from build123d import *

# Parameters (mm, degrees)
SKETCH1_W    = 139.7
SKETCH1_H    = 9.53
BLOCK1_DEPTH = 71.42
SKETCH2_W    = 9.53
SKETCH2_H    = 38.1
BLOCK2_DEPTH = 71.42
SKETCH3_W    = 9.53
SKETCH3_H    = 38.1
BLOCK3_DEPTH = 71.42


with BuildPart() as part:
    # Sketch1 → Block1 (new body)
    with BuildSketch(Plane.XY.offset(-35.71)):
        with Locations((0, 4.765)):
            Rectangle(SKETCH1_W, SKETCH1_H)
    extrude(amount=BLOCK1_DEPTH)

    # Sketch2 → Block2 (add)
    with BuildSketch(Plane.XY.offset(-35.71)):
        with Locations((-55.565, 28.58)):
            Rectangle(SKETCH2_W, SKETCH2_H)
    extrude(amount=BLOCK2_DEPTH)

    # Sketch3 → Block3 (add)
    with BuildSketch(Plane.XY.offset(-35.71)):
        with Locations((55.565, 28.58)):
            Rectangle(SKETCH3_W, SKETCH3_H)
    extrude(amount=BLOCK3_DEPTH)


solid = part.part
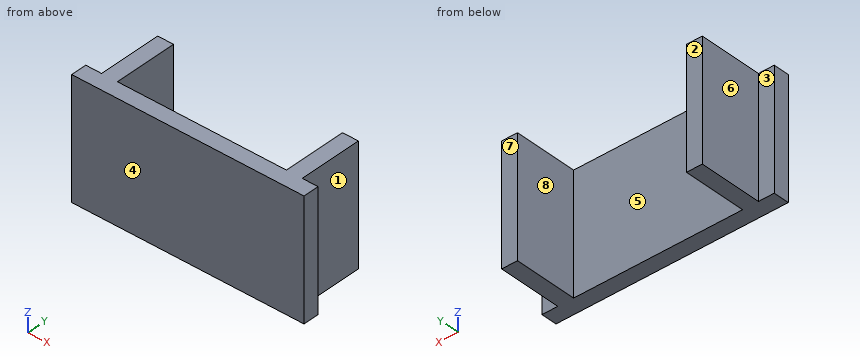
Could you check a few things on this model? Use its own coordinates, in mm. Face numbers are marked on the shaded views. A direction names the side the tool comes from. Coordinates: 2 decimals unless noted, no trailing zeros. Write each loop counter-clockwise with the first axis right and the second up, starting at its lowest first coordinate (ties: lowest second). Pieces come first, ordered by that corner, then holes. Notation, with made-up numbers: (43, -24.75) - (56, -24.75) arc R28 ccw to (56, -3.75) - close; hole circle Ø11 at (25, 2.5). An arc over 180 degrees is marked (long way). Put each result on its own line as item: value. Start each with the question number.
Q1. I'm going to push flat-ended pins straight in: P1, Ø10.5, axis at x = -64.5, z = 9.5, coming from the +Y side; P2, Ø11.5, axis at y = 29.5, z = -7, coming from the -X side; P3, Ø12, axis at y = 18, z = -28, coming from the +X side; P4, Ø7.5, axis at x = 65.5, z = -1, coming from the +Y side. Where does each tip first touch, or does it pass through?
Q2. Thinking about a two-plate mould opening in X: for the marked faces 6, 7 and 8, which applies, pulls with the +X half, pulls with the -X half, needs draft (parallel to the pull), parting line crosses it, or undercut?
Q3. I want a section at C-C on x = 20.5. Write out the boundary of the cut face in (y, z), plus the area to 3 significant figures.
Q4. Which directions (+Z, -Z, +X, -X, +Y, -Y) give clear straight access to the entire face, cutting with the end or side of a thin tool? Please do the marked faces 1, 2, 3, 4 and 5.
Q5. I want a section at A-A on y = 14. Write out the boundary of the cut face in (x, z).
Q6. I want a section at B-B on z = -25. Write out the boundary of the cut face in (x, y), plus the area to 3 significant figures.
Q7. Please list where these lines run through material, in increasing order: L1, parallel to X at y = 43, z = 21; L2, parallel to Y at x = 41, z = -28.
Checks:
1. P1: y = 47.63
1. P2: x = -60.33
1. P3: x = 60.33
1. P4: y = 9.53
2. face 6: pulls with the -X half
2. face 7: needs draft
2. face 8: undercut
3. outline: (0, -35.71) - (9.53, -35.71) - (9.53, 35.71) - (0, 35.71) - close
3. area: 681 mm²
4. face 1: +Z, -Z, +X, +Y
4. face 2: +Z, -Z, +X, -X, +Y
4. face 3: +Z, -Z, -X, +Y
4. face 4: +Z, -Z, +X, -X, -Y
4. face 5: +Z, -Z, +Y
5. outline: (-60.33, -35.71) - (-50.8, -35.71) - (-50.8, 35.71) - (-60.33, 35.71) - close; (50.8, -35.71) - (60.33, -35.71) - (60.33, 35.71) - (50.8, 35.71) - close
6. outline: (-69.85, 0) - (69.85, 0) - (69.85, 9.53) - (60.33, 9.53) - (60.33, 47.63) - (50.8, 47.63) - (50.8, 9.53) - (-50.8, 9.53) - (-50.8, 47.63) - (-60.33, 47.63) - (-60.33, 9.53) - (-69.85, 9.53) - close
6. area: 2,060 mm²
7. L1: -60.33 to -50.8, 50.8 to 60.33
7. L2: 0 to 9.53
